Input: part model. Units: mm. Frame: model coordinates. A direction names the side the tool comes from. Coordinates: 2 decimals unless noted, no trailing zeros. Write each loop counter-clockwise with the first axis right and the second up, starting at its lowest first coordinate (ties: lowest second). Pieces come first, ordered by that corner, then holes.
1) Section query B-B (z = 6). Output: boundary loops of the cut face in (x, y).
2) Pin query (flat end, axial travel): pin 1 Ø10 at (x, y) = (2.5, -2.5) entering from +Z; pin 2 Ø4 at (x, y) = (-13.5, 5) entering from +Z; pin 3 Ø4.5 at (y, z) = (-3.5, 7.5) entering from -X. Return the tip coordinate at first contact, or that it passes through.
3) Section query A-A (x = 13.5). Output: boundary loops of the cut face in (y, z).
4) Draft query along X for faces 3 (the cylindrical face through (12, -5, -1)), 4 (the flat face through (20, 0, 4)), 5 (the flat face through (4, 10, -0.4)). Return one class per face: pulls with the +X half, pulls with the -X half, needs draft (parallel to the pull), parting line crosses it, or undercut.
5) Set-up query: faces 1 (the flat face through (-1, 0, 0)), 2 (the flat face through (22, 0, 4)). Return all of +Z, -Z, +X, -X, +Y, -Y with unobstructed straight access to the full face (end or side cutting, diameter ignored); none if empty.
6) Section query C-C (y = 0). Output: boundary loops of the cut face in (x, z), then the cut area to 3 significant figures.
7) Section query D-D (y = -5). Output: boundary loops of the cut face in (x, z), then the cut area to 3 significant figures.
8) Line query: L1, parallel to Y at x = 13.5, z = -1.8; L2, parallel to Y at x = -13.5, z = -0.7; L3, parallel to X at y = 3, z = -0.75. Output: solid intervals per line, ascending.
from build123d import *

# Parameters (mm, degrees)
SKETCH_1_W                       = 40
SKETCH_1_H                       = 20
SM_BASE_FLANGE_1_DEPTH           = 2
SM_EDGE_FLANGE_1_STRIP_W         = 9.4732
SM_EDGE_FLANGE_1_STRIP_H         = 2
SM_EDGE_FLANGE_1_STRIP_CUT_DEPTH = 20
SM_EDGE_FLANGE_1_DEPTH           = 20
HOLE_WIZARD_M3_2_AT_2_COUNT      = 2
HOLE_WIZARD_M3_2_AT_2_PITCH      = 27
HOLE_WIZARD_M3_1_D               = 3
HOLE_WIZARD_M3_2_2_D             = 3


# Sheet-metal steps are written as plain solids
with BuildPart() as part:
    # Sketch 1 → 基材-凸緣1 (new body)
    with BuildSketch(Plane.XY):
        Rectangle(SKETCH_1_W, SKETCH_1_H)
    extrude(amount=-SM_BASE_FLANGE_1_DEPTH)

    # 邊線-凸緣1 strip (across the edge) → 邊線-凸緣1 strip cut (cut)
    with BuildSketch(Plane(origin=(20, -10, 0), x_dir=(-1, 0, 0), z_dir=(0, 1, 0))):
        with Locations((-4, -1)):
            Rectangle(SM_EDGE_FLANGE_1_STRIP_W, SM_EDGE_FLANGE_1_STRIP_H)
    extrude(amount=SM_EDGE_FLANGE_1_STRIP_CUT_DEPTH, mode=Mode.SUBTRACT)

    # 邊線-凸緣1 section (across the edge) → 邊線-凸緣1 (add)
    with BuildSketch(Plane(origin=(20, -10, 0), x_dir=(-1, 0, 0), z_dir=(0, 1, 0))):
        with BuildLine():
            Line((-2, 0.7366), (-2, 10))
            Line((-2, 10), (0, 10))
            Line((0, 10), (0, 0.7366))
            ThreePointArc((0, 0.7366), (0.215745145, 0.215745145), (0.7366, 0))
            Line((0.7366, 0), (0.7366, -2))
            ThreePointArc((0.7366, -2), (-1.198468417, -1.198468417), (-2, 0.7366))
        make_face()
    extrude(amount=SM_EDGE_FLANGE_1_DEPTH)

    # 草圖11 → Hole Wizard M3 _2 (revolve, cut)
    with BuildSketch(Plane(origin=(-13.5, 5, 0), x_dir=(0, -1, 0), z_dir=(1, 0, 0))):
        Polygon((0, 0), (0, 2), (1.7, 2), (1.7, 1.45), (3.15, 0), align=None)
    hole_wizard_m3_2 = revolve(axis=Axis((-13.5, 5, 6.35), (0, 0, -1)), mode=Mode.SUBTRACT)

    # Hole Wizard M3 _2 at 2: Hole Wizard M3 _2 ×2
    with Locations(*[(i * HOLE_WIZARD_M3_2_AT_2_PITCH, 0, 0) for i in range(1, HOLE_WIZARD_M3_2_AT_2_COUNT)]):
        add(hole_wizard_m3_2, mode=Mode.SUBTRACT)

    # M3 螺紋孔1 (through all)
    with Locations(Plane(origin=(22, 0, 0), x_dir=(0, 0, -1), z_dir=(1, 0, 0))):
        with Locations((-6, 0)):
            Hole(HOLE_WIZARD_M3_1_D / 2)

    # Hole Wizard M3 _2 2 (through all)
    with Locations(Plane(origin=(0, 0, -2), x_dir=(-1, 0, 0), z_dir=(0, 0, -1))):
        with Locations((-13.5, -5), (13.5, -5)):
            Hole(HOLE_WIZARD_M3_2_2_D / 2)


solid = part.part
Answer:
1. outline: (20, -10) - (22, -10) - (22, -1.5) - (20, -1.5) - close; (20, 1.5) - (22, 1.5) - (22, 10) - (20, 10) - close
2. pin 1: stops at z = 0
2. pin 2: stops at z = -1.15
2. pin 3: stops at x = 20
3. outline: (-10, -2) - (-6.5, -2) - (-6.5, 0) - (-10, 0) - close; (-3.5, -2) - (3.3, -2) - (3.3, -1.45) - (1.85, 0) - (-3.5, 0) - close; (6.7, -2) - (10, -2) - (10, 0) - (8.15, 0) - (6.7, -1.45) - close
4. face 3: undercut
4. face 4: pulls with the -X half
4. face 5: needs draft
5. face 1: +Z, -X, +Y, -Y
5. face 2: +Z, -Z, +X, +Y, -Y
6. outline: (-20, -2) - (19.26, -2) arc R2.74 ccw to (22, 0.74) - (22, 4.5) - (20, 4.5) - (20, 0.74) arc R0.74 cw to (19.26, 0) - (-20, 0) - close; (20, 7.5) - (22, 7.5) - (22, 10) - (20, 10) - close
6. area: 96.5 mm2
7. outline: (-20, -2) - (-15, -2) - (-15, 0) - (-20, 0) - close; (-12, -2) - (12, -2) - (12, 0) - (-12, 0) - close; (15, -2) - (19.26, -2) arc R2.74 ccw to (22, 0.74) - (22, 10) - (20, 10) - (20, 0.74) arc R0.74 cw to (19.26, 0) - (15, 0) - close
7. area: 90.5 mm2
8. L1: y = -10 to -6.5, -3.5 to 3.3, 6.7 to 10
8. L2: y = -10 to -6.5, -3.5 to 2.55, 7.45 to 10
8. L3: x = -20 to -14.83, -12.17 to 12.17, 14.83 to 21.56
